Autodesk Inventor part; units mm, degrees
ref_plane "YZ Plane" through (0, 0, 0) normal (1, 0, 0) x (0, 1, 0)
ref_plane "XZ Plane" through (0, 0, 0) normal (0, 1, 0) x (-1, 0, 0)
ref_plane "XY Plane" through (0, 0, 0) normal (0, 0, 1) x (1, 0, 0)
sketch "Sketch1" plane through (0, 0, 0) normal (0, 0, 1) x (1, 0, 0)
  line L0 (38.1, 0) -> (38.1, -3.175)
  line L1 (0, 0) -> (38.1, 0)
  line L2 (38.1, 0) -> (38.1, -158.75)
  line L3 (38.1, -158.75) -> (0, -158.75)
  line L4 (0, -158.75) -> (0, 0)
  circle A0 centre (6.35, -146.05) radius 2.4384
  line L5 (19.05, -158.75) -> (19.05, 0) construction
  circle A1 centre (31.75, -146.05) radius 2.4384
  circle A2 centre (7.6581, -23.6982) radius 2.4384
  circle A3 centre (7.6581, -10.9982) radius 2.4384
  circle A4 centre (30.4419, -10.9982) radius 2.4384
  circle A5 centre (30.4419, -23.6982) radius 2.4384
  line L6 (7.6581, -10.9982) -> (7.6581, -23.6982) construction
  line L7 (31.75, -136.525) -> (6.35, -136.525) construction
  line L8 (6.35, -136.525) -> (6.35, -34.925) construction
  line L9 (6.35, -34.925) -> (31.75, -34.925) construction
  line L10 (31.75, -34.925) -> (31.75, -136.525) construction
  circle A6 centre (19.05, -34.925) radius 2.0828
  circle A7 centre (19.05, -60.325) radius 2.0828
  circle A8 centre (19.05, -85.725) radius 2.0828
  circle A9 centre (19.05, -111.125) radius 2.0828
  circle A10 centre (19.05, -136.525) radius 2.0828
  dimension "d0" = 4.8768
  dimension "d1" = 158.75
  dimension "d2" = 12.7
  dimension "d3" = 12.7
  dimension "d4" = 12.7
  dimension "d5" = 11.3919
  dimension "d6" = 122.3518
  dimension "d7" = 38.1
  dimension "d8" = 25.4
  dimension "d9" = 34.925
  dimension "d10" = 101.6
  dimension "d11" = 4.1656
  dimension "d14" = 25.4
extrude "Extrusion1" add sketch "Sketch1" along normal blind 3.175
properties part number "Support for 9-16 Piston"
For this review, take the finished solid that the model builds, in its own axes (mm). Round coordinates to 2 decimals unless told otherwise and drop trailing zeros. Order: outer loops, then holes, each group sorted by start corner. A loop starts at its lowest first (then second) coordinate and runs counter-clockwise, first axis right, second up. Notation, with made-up numbers: (-39.5, 7) -> (-15.5, 7) arc R23 ccw to (-15.5, 37) -> close; hole circle Ø9 at (81, 71.25). An arc over 180 degrees is marked (long way). Put each result on its own line as item: value.
Q1. Add section A-A on y = -146.05. Write out the cut boundary in (x, z) (3 decimals).
Check result:
outline: (0, 0) -> (3.912, 0) -> (3.912, 3.175) -> (0, 3.175) -> close; (8.788, 0) -> (29.312, 0) -> (29.312, 3.175) -> (8.788, 3.175) -> close; (34.188, 0) -> (38.1, 0) -> (38.1, 3.175) -> (34.188, 3.175) -> close
Q2. For probe 1 along Y at (x, z) = (19.05, 2.1); probe 2 along X at (y, z) = (-146.05, 0.95); probe 3 along Y at (x, z) = (18, 2.9), list the stretches that pass through material, from the lowest coordinate up. Write a range as [from, to].
Check result:
probe 1: [-158.75, -138.61], [-134.44, -113.21], [-109.04, -87.81], [-83.64, -62.41], [-58.24, -37.01], [-32.84, 0]
probe 2: [0, 3.91], [8.79, 29.31], [34.19, 38.1]
probe 3: [-158.75, -138.32], [-134.73, -112.92], [-109.33, -87.52], [-83.93, -62.12], [-58.53, -36.72], [-33.13, 0]
Q3. Add section B-B on x = 19.05. Write out the cut boundary in (y, z) (3 decimals).
Check result:
outline: (-158.75, 0) -> (-138.608, 0) -> (-138.608, 3.175) -> (-158.75, 3.175) -> close; (-134.442, 0) -> (-113.208, 0) -> (-113.208, 3.175) -> (-134.442, 3.175) -> close; (-109.042, 0) -> (-87.808, 0) -> (-87.808, 3.175) -> (-109.042, 3.175) -> close; (-83.642, 0) -> (-62.408, 0) -> (-62.408, 3.175) -> (-83.642, 3.175) -> close; (-58.242, 0) -> (-37.008, 0) -> (-37.008, 3.175) -> (-58.242, 3.175) -> close; (-32.842, 0) -> (0, 0) -> (0, 3.175) -> (-32.842, 3.175) -> close
Q4. Mouldability with a two-part tool opening along X and no side actions: class faces 1 (the flat face through (19, 0, 2)), 2 (the flat face through (0, -80, 2)), 3 (the cylindrical face through (18.6, -58.29, 1.57)) as pulls with the +X half, pulls with the -X half, needs draft (parallel to the pull), parting line crosses it, or undercut.
Check result:
face 1: needs draft
face 2: pulls with the -X half
face 3: undercut
Q5. Add section C-C on z = 1.85. State how many separate pieces and enclosed holes the cut face has, plus the area to 3 significant figures.
Check result:
separate pieces: 1
enclosed holes: 11
area: 5,870 mm2
Q6. Add section D-D on x = 31. Write out the cut boundary in (y, z) (3 decimals).
Check result:
outline: (-158.75, 0) -> (-148.37, 0) -> (-148.37, 3.175) -> (-158.75, 3.175) -> close; (-143.73, 0) -> (-26.072, 0) -> (-26.072, 3.175) -> (-143.73, 3.175) -> close; (-21.325, 0) -> (-13.372, 0) -> (-13.372, 3.175) -> (-21.325, 3.175) -> close; (-8.625, 0) -> (0, 0) -> (0, 3.175) -> (-8.625, 3.175) -> close
